Could you check a few things on this drawing? It's one solid part, dimensions in mm from its lowest x, y, z. A direction names the side the tool comes from. Coordinates: 2 decimals unless noted, no trailing zeros. Write each loop counter-clockwise with the first axis right and the second up, starting at its lowest first coordinate (ties: lowest second). Pieces come first, ordered by that corner, then holes. Notation, with made-up numbers: M -17.5,51 L 32.5,51 A12 ccw 32.5,71 Z; hole C 21.25,50.5 d11. An arc over 180 degrees is marked long. Use a Markdown table: item, result.
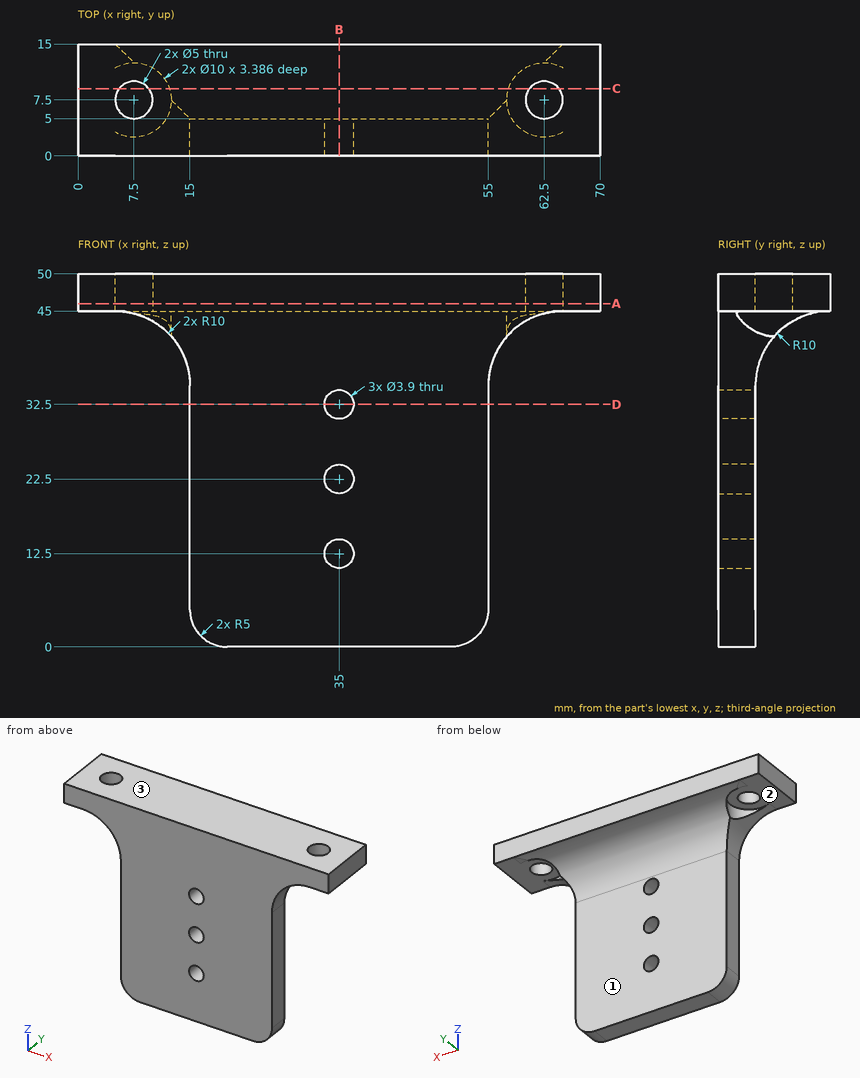
1. I need wall thicknesses on probe 1 along X at (y, z) = (2.1, 12.5); probe 2 along Y at (x, z) = (7, 48); probe 3 along Y at (x, z) = (16, 24). Which ranges of each line are inside material? Lowest first, please.
Answers follow:
| item | result |
|---|---|
| probe 1 | x = 15 to 33.05, 36.95 to 55 |
| probe 2 | y = 0 to 5.05, 9.95 to 15 |
| probe 3 | y = 0 to 5 |
2. Suppose I cut it at C-C on y = 9. Write out the boundary of the cut face in (x, z).
Answers follow:
| item | result |
|---|---|
| outline | M 0,45 L 5.5,45 L 5.5,50 L 0,50 Z; M 9.5,45 L 12.27,45 L 12.27,43 L 57.73,43 L 57.73,45 L 60.5,45 L 60.5,50 L 9.5,50 Z; M 64.5,45 L 70,45 L 70,50 L 64.5,50 Z |
3. Which directions (+Z, -Z, +X, -X, +Y, -Y) give clear straight access to the entire face, cutting with the end or side of a thin tool? Please do the marked faces 1, 2 and 3.
Answers follow:
| item | result |
|---|---|
| face 1 | -Z, +X, -X, +Y |
| face 2 | -Z |
| face 3 | +Z, +X, -X, +Y, -Y |
4. Will these pins go through, and if not, where does the flat tip stop? pin 1 Ø5 at (x, z) = (35, 32.5) entering from +Y; pin 2 Ø5.5 at (y, z) = (3, 22.5) entering from +X; pin 3 Ø5.5 at (y, z) = (2, 18.5) entering from -X.
Answers follow:
| item | result |
|---|---|
| pin 1 | stops at y = 5 |
| pin 2 | stops at x = 55 |
| pin 3 | stops at x = 15 |
5. Suppose I cut it at A-A on z = 46. Write out the boundary of the cut face in (x, y).
Answers follow:
| item | result |
|---|---|
| outline | M 0,0 L 70,0 L 70,15 L 0,15 Z; hole C 7.5,7.5 d5; hole C 62.5,7.5 d5 |
6. Suppose I cut it at B-B on x = 35. State how many separate pieces and enclosed holes the cut face has, and give its area (3 significant figures).
Answers follow:
| item | result |
|---|---|
| separate pieces | 4 |
| enclosed holes | 0 |
| area | 263 mm2 |
7. Suppose I cut it at D-D on z = 32.5. Write out the boundary of the cut face in (x, y).
Answers follow:
| item | result |
|---|---|
| outline | M 15,0 L 33.05,0 L 33.05,5 L 15,5 Z; M 36.95,0 L 55,0 L 55,5 L 36.95,5 Z |
